```python
from build123d import *

# Parameters (mm, degrees)
CROQUIS1_R              = 1.750000001
SALIENTE_EXTRUIR1_DEPTH = 3


with BuildPart() as part:
    # Croquis1 → Saliente-Extruir1 (new body)
    with BuildSketch(Plane(origin=(0, 0, 0), x_dir=(1, 0, 0), z_dir=(0, 1, 0))):
        with BuildLine():
            Line((32.500000027, -77.500000065), (54.196483333, -77.500000065))
            ThreePointArc((54.196483333, -77.500000065), (54.770251601, -76.983361364), (55.496960614, -76.722555719))
            ThreePointArc((55.496960614, -76.722555719), (56.223669627, -76.983361364), (56.797437895, -77.500000065))
            Line((56.797437895, -77.500000065), (170.500000144, -77.500000065))
            Line((170.500000144, -77.500000065), (170.500000144, -76.500000065))
            ThreePointArc((170.500000144, -76.500000065), (174.500000147, -72.500000061), (178.500000151, -76.500000065))
            Line((178.500000151, -76.500000065), (178.500000151, -77.500000065))
            Line((178.500000151, -77.500000065), (181.500000153, -77.500000065))
            Line((181.500000153, -77.500000065), (181.500000153, -137.860356365))
            Line((181.500000153, -137.860356365), (178.718053625, -137.860356365))
            Line((178.718053625, -137.860356365), (178.718053625, -141.000000119))
            Line((178.718053625, -141.000000119), (178.500000151, -141.000000119))
            Line((178.500000151, -141.000000119), (178.500000151, -142.00000012))
            ThreePointArc((178.500000151, -142.00000012), (174.500000147, -146.000000123), (170.500000144, -142.00000012))
            Line((170.500000144, -142.00000012), (170.500000144, -141.000000119))
            Line((170.500000144, -141.000000119), (56.797437895, -141.000000119))
            ThreePointArc((56.797437895, -141.000000119), (56.223669627, -141.516638821), (55.496960614, -141.777444465))
            ThreePointArc((55.496960614, -141.777444465), (54.770251601, -141.516638821), (54.196483333, -141.000000119))
            Line((54.196483333, -141.000000119), (32.500000027, -141.000000119))
            Line((32.500000027, -141.000000119), (32.500000027, -112.000000094))
            ThreePointArc((32.500000027, -112.000000094), (31.025757989, -104.563270659), (30.501093828, -97.000000082))
            ThreePointArc((30.501093828, -97.000000082), (31.025757989, -89.436729506), (32.500000027, -82.000000069))
            Line((32.500000027, -82.000000069), (32.500000027, -77.500000065))
        make_face()
        with Locations(Location((34.000000029, -97.000000082, 0), (0, 0, 270))):
            Circle(CROQUIS1_R, mode=Mode.SUBTRACT)
    extrude(amount=SALIENTE_EXTRUIR1_DEPTH)


solid = part.part
```
Model file for the job. Use its own axes, mm. A direction names the side the tool comes from. Coordinates: 2 decimals unless noted, no trailing zeros. Write each loop counter-clockwise with the first axis right and the second up, starting at its lowest first coordinate (ties: lowest second). Pieces come first, ordered by that corner, then holes. Notation, with made-up numbers: (55, 11) - (104, 11) arc R9 cw to (104, 20) - close; hole circle Ø9 at (-26.75, 4.5). An arc over 180 degrees is marked (long way). One line per question, with ' | ' between items. Start each with the question number.
Q1. Pull direction X, two halves, no side cores. Call faces 6 (the face through (44, 1, 141)), 7 (the face through (113, 1, 77.5)), 8 (the face through (174.6, 1.5, 146)): pulls with the +X half, pulls with the -X half, needs draft (parallel to the pull), parting line crosses it, or undercut.
Q2. Drill centre lines: line 1 (Z direction, x = 153, y = 1.8); line 2 (X direction, y = 1.85, z = 138); line 3 (X direction, y = 0.9, z = 80.5). Where is each one in solid material? Low to high. Write a range as [from, to].
Q3. Cut at B-B, the plane y = 0.6. List the corners of the cut face in (x, z).
Q4. Cut at A-A, the plane x = 34. List the corners of the cut face in (y, z).
Q5. Cut at C-C, the plane x = 110. List the corners of the cut face in (y, z).
Q6. 3-axis set-ups, long thin cutter, end or side, ignore diameter. For faces 1 (the face through (180, 1, 77.5)), 2 (the face through (32.5, 1, 80)), 3 (the face through (32.5, 1, 127)), 4 (the face through (114, 1, 141)), 5 (the face through (180, 1, 137.86)): which of +Z, -Z, +X, -X, +Y, -Y reach the whole face in a straight line?
Q7. Pin check, flat tips, straight feed: pin 1 (1.5 mm diameter, centred on y = 1, z = 139, fed in from +X); pin 2 (1.5 mm diameter, centred on y = 1.5, z = 79, fed in from -X); pin 3 (0.8 mm diameter, centred on y = 1, z = 141.5, fed in from -X). Stop position of each tip, or through.
Answer below:
1) face 6: needs draft | face 7: undercut | face 8: parting line crosses it
2) line 1: [77.5, 141] | line 2: [32.5, 178.72] | line 3: [32.5, 181.5]
3) outline: (30.5, 97) arc R60 ccw to (32.5, 82) - (32.5, 77.5) - (54.2, 77.5) arc R2 ccw to (55.5, 76.72) arc R2 ccw to (56.8, 77.5) - (170.5, 77.5) - (170.5, 76.5) arc R4 ccw to (178.5, 76.5) - (178.5, 77.5) - (181.5, 77.5) - (181.5, 137.86) - (178.72, 137.86) - (178.72, 141) - (178.5, 141) - (178.5, 142) arc R4 ccw to (170.5, 142) - (170.5, 141) - (56.8, 141) arc R2 ccw to (55.5, 141.78) arc R2 ccw to (54.2, 141) - (32.5, 141) - (32.5, 112) arc R60 ccw to start; hole circle Ø3.5 at (34, 97)
4) outline: (0, 77.5) - (3, 77.5) - (3, 95.25) - (0, 95.25) - close; (0, 98.75) - (3, 98.75) - (3, 141) - (0, 141) - close
5) outline: (0, 77.5) - (3, 77.5) - (3, 141) - (0, 141) - close
6) face 1: -Z, +X, +Y, -Y | face 2: -Z, -X, +Y, -Y | face 3: +Z, -X, +Y, -Y | face 4: +Z, +Y, -Y | face 5: +Z, +X, +Y, -Y
7) pin 1: x = 178.72 | pin 2: x = 32.5 | pin 3: x = 54.28
